Design review of the part built by this model. Coordinates are the model's own, in mm. A direction names the side the tool comes from. Give positions to 0.01 mm unless a question says otherwise; leave off trailing zeros. Order: outer loops, then holes, each group sorted by start corner. A loop starts at its lowest first (then second) coordinate and runs counter-clockwise, first axis right, second up. Notation, with made-up numbers: (77.25, 7.5) -> (86.25, 7.5) arc R23 ccw to (86.25, 25.5) -> close; hole circle Ø7 at (-36, 28.25). An arc over 180 degrees is marked (long way). Return JSON: item names as keys, results as strings.
```python
from build123d import *

# Parameters (mm, degrees)
F1_DEPTH = 3.175


# Not quite as in the source:
# - a length typed as a fraction of an inch, garbled in the dataset ("3 / 203.2 mm" for 3/8 in), is restored


with BuildPart() as f1:
    # F0 (on Front) → F1 (new body)
    with BuildSketch(Plane.XZ):
        Polygon((-22.5, -4), (-19.325, -4), (-19.325, -19.325), (-4, -19.325), (-4, -22.5), (0, -22.5), (0, -18), (-18, -18), (-18, 0), (-22.5, 0), align=None)
        Polygon((-22.5, 4), (-22.5, 0), (-18, 0), (-18, 18), (0, 18), (0, 22.5), (-4, 22.5), (-4, 19.325), (-19.325, 19.325), (-19.325, 4), align=None)
        Polygon((0, -18), (0, -22.5), (4, -22.5), (4, -19.325), (19.325, -19.325), (19.325, -4), (22.5, -4), (22.5, 0), (18, 0), (18, -18), align=None)
        Polygon((18, 18), (18, 0), (22.5, 0), (22.5, 4), (19.325, 4), (19.325, 19.325), (4, 19.325), (4, 22.5), (0, 22.5), (0, 18), align=None)
        with BuildLine():
            Line((-18, 18), (-18, 0))
            Line((-18, 0), (0, 0))
            Line((0, 0), (0, 13.25))
            ThreePointArc((0, 13.25), (-1.75, 15), (0, 16.75))
            Line((0, 16.75), (0, 18))
            Line((0, 18), (-18, 18))
        make_face()
        with BuildLine():
            Line((0, 13.25), (0, 0))
            Line((0, 0), (18, 0))
            Line((18, 0), (18, 18))
            Line((18, 18), (0, 18))
            Line((0, 18), (0, 16.75))
            ThreePointArc((0, 16.75), (1.2374368671, 16.2374368671), (1.75, 15))
            ThreePointArc((1.75, 15), (1.2374368671, 13.7625631329), (0, 13.25))
        make_face()
        with BuildLine():
            Line((18, 0), (0, 0))
            Line((0, 0), (0, -13.25))
            ThreePointArc((0, -13.25), (1.2374368671, -13.7625631329), (1.75, -15))
            ThreePointArc((1.75, -15), (1.2374368671, -16.2374368671), (0, -16.75))
            Line((0, -16.75), (0, -18))
            Line((0, -18), (18, -18))
            Line((18, -18), (18, 0))
        make_face()
        with BuildLine():
            Line((0, 0), (-18, 0))
            Line((-18, 0), (-18, -18))
            Line((-18, -18), (0, -18))
            Line((0, -18), (0, -16.75))
            ThreePointArc((0, -16.75), (-1.75, -15), (0, -13.25))
            Line((0, -13.25), (0, 0))
        make_face()
    extrude(amount=F1_DEPTH)


solid = f1.part
```
Item 1: Add section A-A (y = -1). Give the boundary of the cut face in (x, z) (3 decimals).
Result set:
{"outline": "(-22.5, -4) -> (-19.325, -4) -> (-19.325, -19.325) -> (-4, -19.325) -> (-4, -22.5) -> (4, -22.5) -> (4, -19.325) -> (19.325, -19.325) -> (19.325, -4) -> (22.5, -4) -> (22.5, 4) -> (19.325, 4) -> (19.325, 19.325) -> (4, 19.325) -> (4, 22.5) -> (-4, 22.5) -> (-4, 19.325) -> (-19.325, 19.325) -> (-19.325, 4) -> (-22.5, 4) -> close; hole circle Ø3.5 at (0, -15); hole circle Ø3.5 at (0, 15)"}
Item 2: Add section D-D (x = 10). Give the boundary of the cut face in (y, z) (3 decimals).
Result set:
{"outline": "(-3.175, -19.325) -> (0, -19.325) -> (0, 19.325) -> (-3.175, 19.325) -> close"}
Item 3: For pin 1 (1 mm diameter, centred on y = -1.5, z = -20.5, fed in from +X); pin 2 (1 mm diameter, centred on y = -2, z = 14.5, fed in from +X) (3 decimals); pin 3 (1.6 mm diameter, centred on x = -10, y = -2, fed in from -Z) (3 decimals); pin 4 (3 mm diameter, centred on x = -3.5, z = 18, fed in from +Y), all flat-tipped, find the tip position at first contact; note any pin that passes through.
Result set:
{"pin 1": "stops at x = 4", "pin 2": "stops at x = 19.325", "pin 3": "stops at z = -19.325", "pin 4": "stops at y = 0"}
Item 4: Add section B-B (x = -1). Give the boundary of the cut face in (y, z) (3 decimals).
Result set:
{"outline": "(-3.175, -22.5) -> (0, -22.5) -> (0, -16.436) -> (-3.175, -16.436) -> close; (-3.175, -13.564) -> (0, -13.564) -> (0, 13.564) -> (-3.175, 13.564) -> close; (-3.175, 16.436) -> (0, 16.436) -> (0, 22.5) -> (-3.175, 22.5) -> close"}
Item 5: Add section C-C (z = 20). Give the boundary of the cut face in (x, y) (3 decimals), plus the area to 3 significant figures.
Result set:
{"outline": "(-4, -3.175) -> (4, -3.175) -> (4, 0) -> (-4, 0) -> close", "area": "25.4 mm^2"}
Item 6: Machinability: for faces 1 (the face through (-4, -2, -21)), 2 (the face through (12, -2, 19.325)), 3 (the face through (0, -2, 22.5)), 4 (the face through (12, -2, -19.325)), 5 (the face through (-19.325, -2, 12)), which of the approach directions +Z, -Z, +X, -X, +Y, -Y give a long, thin tool a straight path to every point of the face, cutting with its end or side? Answer none if there is none.
Result set:
{"face 1": "-Z, -X, +Y, -Y", "face 2": "+Z, +X, +Y, -Y", "face 3": "+Z, +X, -X, +Y, -Y", "face 4": "-Z, +X, +Y, -Y", "face 5": "+Z, -X, +Y, -Y"}
Item 7: Wall thickness on L1, parallel to Z at x = -10, y = -2.4 (3 decimals); L2, parallel to Z at x = -0.5, y = -2: over which ranges is each line inside the solid? List them lowest first. Write a range as [from, to].
Result set:
{"L1": "z = [-19.325, 19.325]", "L2": "z = [-22.5, -16.68], [-13.32, 13.32], [16.68, 22.5]"}
